Autodesk Inventor part; units mm, degrees
ref_plane "YZ Plane" through (0, 0, 0) normal (1, 0, 0) x (0, 1, 0)
ref_plane "XZ Plane" through (0, 0, 0) normal (0, 1, 0) x (-1, 0, 0)
ref_plane "XY Plane" through (0, 0, 0) normal (0, 0, 1) x (1, 0, 0)
sketch "Sketch1" plane through (0, 0, 0) normal (0, 1, 0) x (-1, 0, 0)
  point P0 (0, 0)
sketch "Sketch2" plane through (0, 0, 0) normal (0, 1, 0) x (-1, 0, 0)
  line L0 (0, 0) -> (16, 0)
  line L1 (16, 0) -> (16, -16)
  line L2 (16, -16) -> (0, -16)
  line L3 (0, -16) -> (0, 0)
  line L4 (0, 0) -> (0, -8)
  dimension "d1" = 16
  dimension "d2" = 16
extrude "Extrusion1" add sketch "Sketch2" along normal blind 16
sketch "Sketch3" plane through (0, 0, 0) normal (0, -1, 0) x (1, 0, 0)
  line L0 (-16, 0) -> (0, 0)
  line L1 (-16, -16) -> (-16, 0)
  line L2 (0, 0) -> (0, -16)
  line L3 (-16, -8) -> (0, -8)
  line L4 (-16, -8) -> (-16, -9.8)
  line L5 (0, -16) -> (0, -14.2)
  line L6 (0, -14.2) -> (-16, -9.8)
  line L7 (-8, -12) -> (-1.7327, -13.7235)
  line L8 (-1.7327, -13.7235) -> (-1.2135, -12)
  line L9 (-1.2135, -12) -> (-13.7482, -8.553)
  line L10 (-13.7482, -8.553) -> (-14.7865, -12)
  line L11 (-14.7865, -12) -> (-2.3425, -15.7481)
  line L12 (-2.3425, -15.7481) -> (-1.7327, -13.7235)
  line L13 (-16, -8) -> (-16, -6.2)
  line L14 (0, 0) -> (0, -1.8)
  line L15 (0, -1.8) -> (-16, -6.2)
  line L16 (-8, -4) -> (-14.2673, -5.7235)
  line L17 (-14.2673, -5.7235) -> (-13.7901, -7.4591)
  line L18 (-13.7901, -7.4591) -> (-1.2554, -4.0121)
  line L19 (-13.7901, -7.4591) -> (-14.7446, -3.9879)
  line L20 (-14.7446, -3.9879) -> (-2.2099, -0.5409)
  line L21 (-2.2099, -0.5409) -> (-1.2554, -4.0121)
  dimension "d28" = 1.8
  dimension "d31" = 1.8
  dimension "d32" = 13
  dimension "d33" = 3.6
  dimension "d34" = 1.8
  dimension "d35" = 1.8
  dimension "d37" = 1.8
  dimension "d38" = 13
  dimension "d42" = 3.6
  dimension "d43" = 13
extrude "Extrusion2" cut sketch "Sketch3" against normal blind 13 contours L19 L20 L21 L15 | L15 L21 L18 L17 | L10 L9 L8 L6 | L6 L12 L11 L10
properties part number "pawn-2"
Here's how the part is built. I have some questions about the finished solid (model axes, mm). A direction names the side the tool comes from. Give positions to 0.01 mm unless a question says otherwise; leave off trailing zeros. Order: outer loops, then holes, each group sorted by start corner. A loop starts at its lowest first (then second) coordinate and runs counter-clockwise, first axis right, second up. Notation, with made-up numbers: (52, 34.5) - (76, 34.5) arc R4 ccw to (76, 41.5) - close; hole circle Ø4 at (72.25, -18). An arc over 180 degrees is marked (long way). Answer as a JSON object with one key per item and string values. Group by question number.
Item 1: For P1, Ø8, axis at x = -7.5, y = 5, coming from the +Z side; P2, Ø2, axis at x = -6.5, z = -3.5, coming from the -Y side, each with a flat end and sliding along its axis, tell me the tip position at first contact or that it passes through.
Item 2: Please list where these lines run through material, in increasing order: probe 1 along Z at (x, y) = (-12.25, 11) (3 decimals); probe 2 along Z at (x, y) = (-6.25, 12.5); probe 3 along Y at (x, z) = (-13.25, -9.5).
Item 3: Which directions (+Z, -Z, +X, -X, +Y, -Y) give clear straight access to the entire face, cutting with the end or side of a thin tool? Please do faces 1 (the flat face through (-8.65, 6.41, -13.85)), 2 (the flat face through (-8, 16, -8)).
Item 4: If we section it at B-B on x = -13.25: Please give me the cut outline in (y, z), and give its area (3 significant figures).
Item 5: If we section it at A-A on y = 6: Please give me the cut outline in (x, z).
Item 6: If we section it at D-D on x = -8: Please give me the cut outline in (y, z).
Item 7: If we section it at C-C on z = -14.75: Please give me the cut outline in (x, y).
Item 8: If we mould it in two halves opening along Z, with no side actions, what happens to faces 3 (the flat face through (-8, 13, -4)), 4 (the flat face through (0, 8, -8)), 5 (the flat face through (-8, 8, 0))? For each: pulls with the +Z half, pulls with the -Z half, needs draft (parallel to the pull), parting line crosses it, or undercut.
Result set:
{
 "1": {"P1": "z = 0", "P2": "y = 13"},
 "2": {"probe 1": "-16 to -12.764, -8.965 to -7.036, -3.302 to 0", "probe 2": "-16 to -14.57, -10.61 to -5.39, -1.65 to 0", "probe 3": "13 to 16"},
 "3": {"face 1": "-Y", "face 2": "+Z, -Z, +X, -X, +Y"},
 "4": {"outline": "(0, -16) - (16, -16) - (16, 0) - (0, 0) - (0, -3.58) - (13, -3.58) - (13, -7.31) - (0, -7.31) - (0, -8.69) - (13, -8.69) - (13, -12.46) - (0, -12.46) - close", "area": "158 mm²"},
 "5": {"outline": "(-16, -16) - (0, -16) - (0, 0) - (-16, 0) - close; hole (-14.79, -12) - (-2.34, -15.75) - (-1.73, -13.72) - (-1.21, -12) - (-13.75, -8.55) - close; hole (-14.74, -3.99) - (-14.27, -5.72) - (-13.79, -7.46) - (-1.26, -4.01) - (-2.21, -0.54) - close"},
 "6": {"outline": "(0, -16) - (16, -16) - (16, 0) - (0, 0) - (0, -2.13) - (13, -2.13) - (13, -5.87) - (0, -5.87) - (0, -10.13) - (13, -10.13) - (13, -14.04) - (0, -14.04) - close"},
 "7": {"outline": "(-16, 0) - (-5.66, 0) - (-5.66, 13) - (-2.04, 13) - (-2.04, 0) - (0, 0) - (0, 16) - (-16, 16) - close"},
 "8": {"face 3": "undercut", "face 4": "needs draft", "face 5": "pulls with the +Z half"}
}
